Build history of the part. All positions in model axes, mm. A direction names the side the tool comes from. Give positions to 0.01 mm unless a question says otherwise; leave off trailing zeros. Loops run counter-clockwise (first coordinate to the right, second up) from the corner with the lowest first, then second, coordinate; pieces in that order, holes last. Notation, with made-up numbers: M -24,-23.5 L 2,-23.5 A21 ccw 2,3.5 Z; hole C 89,26 d6. An arc over 180 degrees is marked long. Answer in a Markdown table with one row per item. Add a question column.
```python
from build123d import *

# Parameters (mm, degrees)
CROQUIS1_W              = 70
CROQUIS1_H              = 110
CROQUIS1_W_2            = 13.66965824
CROQUIS1_H_2            = 19.532598364
SALIENTE_EXTRUIR1_DEPTH = 7.9375
CROQUIS2_W              = 97.0625
CROQUIS2_H              = 70
SALIENTE_EXTRUIR2_DEPTH = 7.9375
SALIENTE_EXTRUIR3_DEPTH = 7.9375


with BuildPart() as part:
    # Croquis1 → Saliente-Extruir1 (new body)
    # profile 1 of 2: a face of its own
    with BuildSketch(Plane(origin=(0, 0, 0), x_dir=(0, 0, -1), z_dir=(1, 0, 0))):
        with Locations((0, 25)):
            Rectangle(CROQUIS1_W, CROQUIS1_H)
        with BuildLine():
            Line((6.83482912, 65), (6.83482912, -10))
            ThreePointArc((6.83482912, -10), (0, -16.83482912), (-6.83482912, -10))
            Line((-6.83482912, -10), (-6.83482912, 65))
            ThreePointArc((-6.83482912, 65), (0, 71.83482912), (6.83482912, 65))
        make_face(mode=Mode.SUBTRACT)
    # profile 2 of 2: a face of its own
    with BuildSketch(Plane(origin=(0, 0, 0), x_dir=(0, 0, -1), z_dir=(1, 0, 0))):
        with Locations((0, 27.5)):
            Rectangle(CROQUIS1_W_2, CROQUIS1_H_2)
    extrude(amount=SALIENTE_EXTRUIR1_DEPTH)

    # Croquis2 → Saliente-Extruir2 (add)
    with BuildSketch(Plane.XZ.offset(30)):
        with Locations((56.46875, 0)):
            Rectangle(CROQUIS2_W, CROQUIS2_H)
        with BuildLine():
            ThreePointArc((30, -6.640349162), (23.359650838, 0), (30, 6.640349162))
            Line((30, 6.640349162), (90, 6.640349162))
            ThreePointArc((90, 6.640349162), (96.640349162, 0), (90, -6.640349162))
            Line((90, -6.640349162), (30, -6.640349162))
        make_face(mode=Mode.SUBTRACT)
    extrude(amount=-SALIENTE_EXTRUIR2_DEPTH)

    # Croquis3 → Saliente-Extruir3 (add)
    with BuildSketch(Plane(origin=(0, 0, 35), x_dir=(-1, 0, 0), z_dir=(0, 0, -1))):
        Polygon((0, 45.166428926), (-75.166428926, -30), (0, -30), align=None)
    extrude(amount=SALIENTE_EXTRUIR3_DEPTH)


solid = part.part
```
(1) Slice it at A-A, the plane z = 0. Give the cut face in (x, y), then the cut area to 3 significant figures.
(2) Slice it at C-C, the plane y = 10. Give the cut face in (x, z).
(3) Slice it at B-B, the plane x = 84.5. Give the cut face in (y, z).
(4) Slice it at D-D, the plane z = -20. Give the cut face in (x, y), then the cut area to 3 significant figures.
(5) Tool access for faces 5 (the cylindrical face through (96.64, -26.09, 0.15)), 6 (the cylindrical face through (3.913, 71.833, 0.15)), 7 (the flat face through (56, -22.062, -7)): list every direction of +Z, -Z, +X, -X, +Y, -Y with a clear straight run to the whole face (end or side of a thin tool).
(6) Wall check: line 1 (Y direction, x = 18.5, z = 16); line 2 (X direction, y = 65.5, z = 26.5); line 3 (Z direction, x = 19, y = 5.5). Give the ranges that are in metal, low to high.
(7) Pull direction X, two halves, no side cores. Call faces 1 (the flat face through (60, -26, -6.64)), 2 (the cylindrical face through (23.36, -26.09, -0.15)), 3 (the flat face through (7.938, 30, 0)), 4 (the flat face through (4, 80, 0)): +X half, -X half, draft (parallel to the pull), parting line (faces both ways), or undercut.
(8) Pin check, flat tips, straight feed: pin 1 (8 mm diameter, centred on x = 84, z = 4, fed in from +Y); pin 2 (2 mm diameter, centred on y = 11.5, z = 8.5, fed in from +X); pin 3 (5 mm diameter, centred on x = 35, y = 13, fed in from -Z). Stop position of each tip, or through.
Solution:
| question | item | result |
|---|---|---|
| 1 | outline | M 0,-30 L 23.36,-30 L 23.36,-22.06 L 7.94,-22.06 L 7.94,-16.83 L 0,-16.83 Z; M 0,17.73 L 7.94,17.73 L 7.94,37.27 L 0,37.27 Z; M 0,71.83 L 7.94,71.83 L 7.94,80 L 0,80 Z; M 96.64,-30 L 105,-30 L 105,-22.06 L 96.64,-22.06 Z |
| 1 | area | 513 mm^2 |
| 2 | outline | M 0,-35 L 7.94,-35 L 7.94,-6.83 L 0,-6.83 Z; M 0,6.83 L 7.94,6.83 L 7.94,27.06 L 35.17,27.06 L 35.17,35 L 0,35 Z |
| 3 | outline | M -30,-35 L -22.06,-35 L -22.06,-6.64 L -30,-6.64 Z; M -30,6.64 L -22.06,6.64 L -22.06,35 L -30,35 Z |
| 4 | outline | M 0,-30 L 105,-30 L 105,-22.06 L 7.94,-22.06 L 7.94,80 L 0,80 Z |
| 4 | area | 1,640 mm^2 |
| 5 | face 5 | +Y, -Y |
| 5 | face 6 | +X, -X |
| 5 | face 7 | -Z, +X, +Y |
| 6 | line 1 | -30 to -22.06 |
| 6 | line 2 | 0 to 7.94 |
| 6 | line 3 | 27.06 to 35 |
| 7 | face 1 | undercut |
| 7 | face 2 | undercut |
| 7 | face 3 | +X half |
| 7 | face 4 | draft |
| 8 | pin 1 | y = -22.06 |
| 8 | pin 2 | x = 7.94 |
| 8 | pin 3 | z = 27.06 |
